Check sheet for the modelled part. Datum: model origin and axes. Units: mm. A direction names the side the tool comes from. Round coordinates to 2 decimals unless told otherwise and drop trailing zeros. Write each loop counter-clockwise with the first axis right and the second up, starting at its lowest first coordinate (ties: lowest second). Pieces come first, ordered by that corner, then holes.
Item 1: Material ranges on line 1 (X direction, y = 1, z = 27); line 2 (X direction, y = 10.25, z = -10.5); line 3 (X direction, y = 11.05, z = 10.5), recorded low to high.
Item 2: Cross-section at B-B on y = 9.75. Count the separate pieces of the cut face and the enclosed holes in it, plus the area to 3 significant figures.
Item 3: Go/stop test with flat-tipped pins: pin 1 Ø14 at (x, z) = (19.5, -7) entering from -Y; pin 2 Ø2 at (x, z) = (28, -27) entering from +Y; pin 3 Ø8 at (x, z) = (4, -19) entering from +Y; pin 4 Ø3 at (x, z) = (20.5, -27.5) entering from +Y. Record where each tip stops, or that it passes through.
Item 4: Tool access check on faces 4 (the flat face through (12, 9, -11)), 5 (the flat face through (15.8, 12, 6.5)), 6 (the flat face through (24, 14.5, 2.1)). Record the directions out of +Z, -Z, +X, -X, +Y, -Y that give a thin tool (end or side, any length) a straight path to the whole face; none if there is none.
Item 5: Release check for a two-part mould opening along X. For faces 1 (the conical face through (11.306, 9.146, -9.101)), 2 (the cylindrical face through (1.203, 1.232, 29.859)), 3 (the flat face through (12, 9, 10)) record: +X half, -X half, draft (parallel to the pull), parting line (faces both ways), or undercut.
Item 6: Cross-section at A-A on z = -1. Enter the section's corners in (x, y), plus the area to 3 significant figures.
Item 7: Cross-section at C-C on x = 20.5. Enter the section's corners in (y, z), plus the area to 3 significant figures.
from build123d import *

# Parameters (mm, degrees)
EXTRUDE_1_DEPTH                      = 32
SKETCH_2_R                           = 1.75
CUT_EXTRUDE_1_DEPTH                  = 48.010637094
PATTERN_LINEAR_1_COUNT               = 2
PATTERN_LINEAR_1_PITCH               = 24
PATTERN_LINEAR_1_COUNT_DIR2          = 2
PATTERN_LINEAR_1_PITCH_DIR2          = 54
FILLET_1_R                           = 4
FILLET_3_R                           = 6
FILLET_5_R                           = 4
SKETCH_4_W                           = 10
SKETCH_4_H                           = 10
CUT_EXTRUDE_3_DEPTH                  = 48.010637094
FILLET_6_R                           = 2
SKETCH_3_R                           = 2.5
SKETCH_3_R_2                         = 1
EXTRUDE_3_DEPTH                      = 3
CHAMFER_3_SIZE                       = 1.75
CHAMFER_3_SIZE_2                     = 3.031088913
PATTERN_LINEAR_5_COUNT               = 2
PATTERN_LINEAR_5_PITCH               = 12.5
PATTERN_LINEAR_5_COUNT_DIR2          = 2
PATTERN_LINEAR_5_PITCH_DIR2          = 21
CHAMFER_3_OF_PATTERN_LINEAR_5_SIZE   = 1.75
CHAMFER_3_OF_PATTERN_LINEAR_5_SIZE_2 = 3.031088913
CUT_EXTRUDE_5_DEPTH                  = 1
CHAMFER_4_SIZE                       = 1


with BuildPart() as part:
    # Эскиз1 → Бобышка-Вытянуть1 (new body)
    with BuildSketch(Plane(origin=(0, 0, 0), x_dir=(0, 0, -1), z_dir=(1, 0, 0))):
        Polygon((-31, 0), (-20, 0), (-15.632357189, 12), (15.632357189, 12), (20, 0), (31, 0), (31, 2.5), (21.750518846, 2.5), (17.200890917, 15), (-17.200890917, 15), (-21.750518846, 2.5), (-31, 2.5), align=None)
    extrude(amount=EXTRUDE_1_DEPTH)

    # Эскиз2 → Вырез-Вытянуть1 (cut, through all)
    with BuildSketch(Plane.XZ):
        with Locations(Location((4, 27, 0), (0, 0, 270))):
            Circle(SKETCH_2_R)
    cut_extrude_1 = extrude(amount=-CUT_EXTRUDE_1_DEPTH, mode=Mode.SUBTRACT)

    # Линейный массив1: Cut-Extrude 1 2 × 2
    with Locations(*[(i * PATTERN_LINEAR_1_PITCH, 0, -j * PATTERN_LINEAR_1_PITCH_DIR2) for i in range(PATTERN_LINEAR_1_COUNT) for j in range(PATTERN_LINEAR_1_COUNT_DIR2) if (i, j) != (0, 0)]):
        add(cut_extrude_1, mode=Mode.SUBTRACT)

    # Скругление1
    fillet_1_edges = [part.edges().sort_by_distance(p)[0] for p in [
        (0, 1.25, -31),
        (0, 1.25, 31),
        (32, 1.25, -31),
        (32, 1.25, 31),
    ]]
    fillet(fillet_1_edges, radius=FILLET_1_R)

    # Скругление3
    fillet_3_edges = [part.edges().sort_by_distance(p)[0] for p in [
        (16, 15, 17.200890917),
        (16, 15, -17.200890917),
    ]]
    fillet(fillet_3_edges, radius=FILLET_3_R)

    # Скругление5
    fillet_5_edges = [part.edges().sort_by_distance(p)[0] for p in [
        (16, 2.5, 21.750518846),
        (16, 2.5, -21.750518846),
        (16, 0, -20),
        (16, 0, 20),
    ]]
    fillet(fillet_5_edges, radius=FILLET_5_R)

    # Эскиз4 → Вырез-Вытянуть3 (cut, through all)
    with BuildSketch(Plane(origin=(0, 15, 0), x_dir=(1, 0, 0), z_dir=(0, 1, 0))):
        with Locations((13.5, 0)):
            Rectangle(SKETCH_4_W, SKETCH_4_H)
    extrude(amount=-CUT_EXTRUDE_3_DEPTH, mode=Mode.SUBTRACT)

    # Скругление6
    fillet_6_edges = [part.edges().sort_by_distance(p)[0] for p in [
        (16, 12, -15.632357189),
        (16, 12, 15.632357189),
    ]]
    fillet(fillet_6_edges, radius=FILLET_6_R)

    # Эскиз3 → Бобышка-Вытянуть3 (add)
    with BuildSketch(Plane.XZ.offset(-12)):
        with Locations(Location((26, 10.5, 0), (0, 0, 90))):
            Circle(SKETCH_3_R)
        with Locations(Location((26, 10.5, 0), (0, 0, 270))):
            Circle(SKETCH_3_R_2, mode=Mode.SUBTRACT)
    extrude_3 = extrude(amount=EXTRUDE_3_DEPTH)

    # Фаска3
    # the kernel refuses this chamfer: 3.031088913, 1.75 mm, written as the material it adds along each edge
    with BuildSketch(Plane(origin=(26, 12, 10.5), x_dir=(0, 0, 1), z_dir=(1, 0, 0))) as chamfer_3_piece_1_section:
        Polygon((2.5 + CHAMFER_3_SIZE, 0), (2.5, CHAMFER_3_SIZE_2), (2.5, 0), align=None)
    chamfer_3_piece_1 = revolve(axis=Axis((26, 12, 10.5), (0, -1, 0)), mode=Mode.PRIVATE)
    chamfer_3_piece_1 = split(chamfer_3_piece_1, bisect_by=Plane(origin=(26, 9, 7.119181545), z_dir=(0, 1, 0)), keep=Keep.TOP, mode=Mode.PRIVATE)
    add(chamfer_3_piece_1)

    # Линейный массив5: Extrude 3 2 × 2
    with Locations(*[(-i * PATTERN_LINEAR_5_PITCH, 0, -j * PATTERN_LINEAR_5_PITCH_DIR2) for i in range(PATTERN_LINEAR_5_COUNT) for j in range(PATTERN_LINEAR_5_COUNT_DIR2) if (i, j) != (0, 0)]):
        add(extrude_3)

    # Фаска3 of Линейный массив5
    # the kernel refuses this chamfer: 3.031088913, 1.75 mm, written as the material it adds along each edge
    with BuildSketch(Plane(origin=(26, 12, -10.5), x_dir=(0, 0, 1), z_dir=(1, 0, 0))) as chamfer_3_of_pattern_linear_5_piece_1_section:
        Polygon((2.5 + CHAMFER_3_OF_PATTERN_LINEAR_5_SIZE, 0), (2.5, CHAMFER_3_OF_PATTERN_LINEAR_5_SIZE_2), (2.5, 0), align=None)
    chamfer_3_of_pattern_linear_5_piece_1 = revolve(axis=Axis((26, 12, -10.5), (0, -1, 0)), mode=Mode.PRIVATE)
    chamfer_3_of_pattern_linear_5_piece_1 = split(chamfer_3_of_pattern_linear_5_piece_1, bisect_by=Plane(origin=(26, 9, -13.880818454), z_dir=(0, 1, 0)), keep=Keep.TOP, mode=Mode.PRIVATE)
    add(chamfer_3_of_pattern_linear_5_piece_1)
    with BuildSketch(Plane(origin=(13.5, 12, 10.5), x_dir=(0, 0, 1), z_dir=(1, 0, 0))) as chamfer_3_of_pattern_linear_5_piece_2_section:
        Polygon((2.5 + CHAMFER_3_OF_PATTERN_LINEAR_5_SIZE, 0), (2.5, CHAMFER_3_OF_PATTERN_LINEAR_5_SIZE_2), (2.5, 0), align=None)
    chamfer_3_of_pattern_linear_5_piece_2 = revolve(axis=Axis((13.5, 12, 10.5), (0, -1, 0)), mode=Mode.PRIVATE)
    chamfer_3_of_pattern_linear_5_piece_2 = split(chamfer_3_of_pattern_linear_5_piece_2, bisect_by=Plane(origin=(13.5, 9, 7.119181545), z_dir=(0, 1, 0)), keep=Keep.TOP, mode=Mode.PRIVATE)
    add(chamfer_3_of_pattern_linear_5_piece_2)
    with BuildSketch(Plane(origin=(13.5, 12, -10.5), x_dir=(0, 0, 1), z_dir=(1, 0, 0))) as chamfer_3_of_pattern_linear_5_piece_3_section:
        Polygon((2.5 + CHAMFER_3_OF_PATTERN_LINEAR_5_SIZE, 0), (2.5, CHAMFER_3_OF_PATTERN_LINEAR_5_SIZE_2), (2.5, 0), align=None)
    chamfer_3_of_pattern_linear_5_piece_3 = revolve(axis=Axis((13.5, 12, -10.5), (0, -1, 0)), mode=Mode.PRIVATE)
    chamfer_3_of_pattern_linear_5_piece_3 = split(chamfer_3_of_pattern_linear_5_piece_3, bisect_by=Plane(origin=(13.5, 9, -13.880818454), z_dir=(0, 1, 0)), keep=Keep.TOP, mode=Mode.PRIVATE)
    add(chamfer_3_of_pattern_linear_5_piece_3)

    # Эскиз12 → Вырез-Вытянуть5 (cut)
    with BuildSketch(Plane(origin=(0, 15, 0), x_dir=(1, 0, 0), z_dir=(0, 1, 0))):
        Polygon((19.5, 0), (28.56307787, -4.226182617), (26.940798358, 0), (28.56307787, 4.226182617), align=None)
    extrude(amount=-CUT_EXTRUDE_5_DEPTH, mode=Mode.SUBTRACT)

    # Фаска4
    chamfer_4_edges = [part.edges().sort_by_distance(p)[0] for p in [
        (13.5, 12, 5),
        (8.5, 12, 0),
        (13.5, 12, -5),
        (18.5, 12, 0),
    ]]
    chamfer(chamfer_4_edges, length=CHAMFER_4_SIZE)


solid = part.part
Response values:
1. line 1: x = 0 to 2.25, 5.75 to 26.25, 29.75 to 32
1. line 2: x = 10.26 to 12.5, 14.5 to 16.74, 22.76 to 25, 27 to 29.24
1. line 3: x = 9.8 to 12.5, 14.5 to 17.2, 22.3 to 25, 27 to 29.7
2. separate pieces: 6
2. enclosed holes: 4
2. area: 267 mm2
3. pin 1: stops at y = 9
3. pin 2: passes through
3. pin 3: stops at y = 14.66
3. pin 4: stops at y = 2.5
4. face 4: +X, -X, -Y
4. face 5: -Y
4. face 6: +Y
5. face 1: undercut
5. face 2: -X half
5. face 3: draft
6. outline: (0, 12) - (7.5, 12) - (8.5, 13) - (8.5, 15) - (0, 15) - close; (18.5, 13) - (19.5, 12) - (32, 12) - (32, 15) - (27.32, 15) - (27.32, 14) - (21.64, 14) - (21.64, 15) - (18.5, 15) - close
6. area: 59.3 mm2
7. outline: (0, -31) - (2.5, -31) - (2.5, -24.55) arc R4 cw to (5.13, -20.79) - (11.05, -18.64) arc R6 ccw to (15, -13) - (15, -0.47) - (14, -0.47) - (14, 0.47) - (15, 0.47) - (15, 13) arc R6 ccw to (11.05, 18.64) - (5.13, 20.79) arc R4 cw to (2.5, 24.55) - (2.5, 31) - (0, 31) - (0, 22.8) arc R4 ccw to (2.63, 19.04) - (10.68, 16.11) arc R2 cw to (12, 14.23) - (12, -14.23) arc R2 cw to (10.68, -16.11) - (2.63, -19.04) arc R4 ccw to (0, -22.8) - close
7. area: 208 mm2
